Model file for the job. Use its own axes, mm. Face numbers are marked on the shaded views. A direction names the side the tool comes from. Round coordinates to 2 decimals unless told otherwise and drop trailing zeros. Loops run counter-clockwise (first coordinate to the right, second up) from the corner with the lowest first, then second, coordinate; pieces in that order, holes last. Notation, with made-up numbers: M -34.5,3.25 L -16.5,3.25 A21 cw -16.5,29.25 Z; hole C 22.25,-19 d6. An arc over 180 degrees is marked long. Use a Markdown table: item, result. Add a question column.
Item 1: Saw through at D-D on x = 30. Write the cut outline in (y, z), then the cut area to 3 significant figures.
Item 2: Saw through at C-C on z = 26. Write the cut outline in (x, y).
Item 3: Saw through at A-A on x = -22. Write the cut outline in (y, z), then the cut area to 3 significant figures.
Item 4: Saw through at B-B on y = 5.25. Give the number of separate pieces and of enclosed holes in the cut face, then the cut area to 3 significant figures.
Item 5: Pin check, flat tips, straight feed: P1, Ø2, axis at y = 6, z = 23.5, coming from the +X side; P2, Ø5, axis at x = 35, y = 1, coming from the -Z side; P3, Ø3, axis at x = 39.59, z = 45.61, coming from the -Y side; P4, Ø4.5, axis at x = 0, z = 0, coming from the +Y side. Stop position of each tip, or through.
Item 6: Tool access for the marked faces 4 and 5: list every direction of +Z, -Z, +X, -X, +Y, -Y with a clear straight run to the whole face (end or side of a thin tool).
Item 7: Two-plate mould, pull along X, no slides. Class the marked faces 1, 2 and 3: +X half, -X half, draft (parallel to the pull), parting line (faces both ways), or undercut.
Item 8: Wall check: L1, parallel to X at y = 7.5, z = 1.5; L2, parallel to Y at x = -20.5, z = -2.5; L3, parallel to X at y = 5.25, z = 45. Give the ranges that are in metal, low to high. Write a range as from..to.
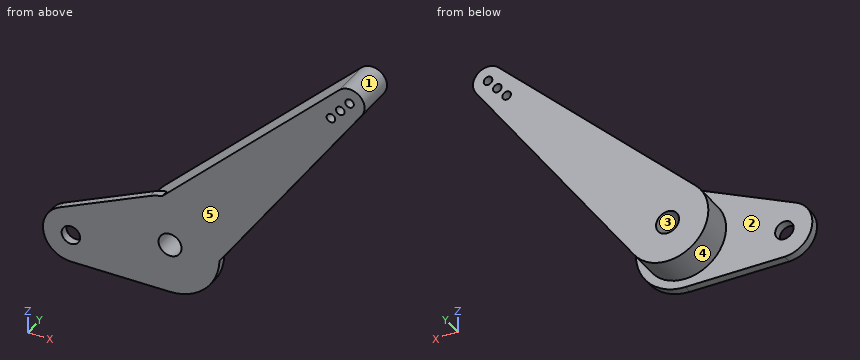
```python
from build123d import *

# Parameters (mm, degrees)
ESQUISSE1_R             = 2.675
ESQUISSE1_R_2           = 2.15
BOSS_EXTRU_1_DEPTH      = 2
BOSS_EXTRU_2_DEPTH      = 7.5
BOSS_EXTRU_2_DEPTH_BACK = 2
ESQUISSE2_R             = 2.675
ESQUISSE2_R_2           = 1


with BuildPart() as part:
    # Esquisse1 → Boss.-Extru.1 (new body)
    with BuildSketch(Plane(origin=(0, 0, 0), x_dir=(1, 0, 0), z_dir=(0, 1, 0))):
        with BuildLine():
            Line((0, 11.5), (-23.064258063, 11.5))
            ThreePointArc((-23.064258063, 11.5), (-29.416702021, 6.377118644), (-25.755971605, -0.916475151))
            Line((-25.755971605, -0.916475151), (-4.76226242, -10.467609882))
            ThreePointArc((-4.76226242, -10.467609882), (11.23893931, -2.436440678), (0, 11.5))
        make_face()
        with Locations(Location((0, 0, 0), (0, 0, 270))):
            Circle(ESQUISSE1_R, mode=Mode.SUBTRACT)
        with Locations(Location((-23.064258063, 5, 0), (0, 0, 270))):
            Circle(ESQUISSE1_R_2, mode=Mode.SUBTRACT)
    extrude(amount=BOSS_EXTRU_1_DEPTH)

    # Esquisse2 → Boss.-Extru.2 (add, two sides: drawn at the far end of the back side and taken through both)
    with BuildSketch(Plane(origin=(0, 2, 0), x_dir=(1, 0, 0), z_dir=(0, 1, 0)).offset(-BOSS_EXTRU_2_DEPTH_BACK)):
        with BuildLine():
            Line((7.728498539, 5.524519013), (44.604848398, -46.063468165))
            ThreePointArc((44.604848398, -46.063468165), (44.052017955, -50.741773707), (39.342439126, -50.632085515))
            Line((39.342439126, -50.632085515), (-6.555183772, -6.876013796))
            ThreePointArc((-6.555183772, -6.876013796), (-6.227958764, 7.173738888), (7.728498539, 5.524519013))
        make_face()
        with Locations(Location((0, 0, 0), (0, 0, 270))):
            Circle(ESQUISSE2_R, mode=Mode.SUBTRACT)
        with Locations(Location((41.757506831, -48.098817275, 0), (0, 0, 270))):
            Circle(ESQUISSE2_R_2, mode=Mode.SUBTRACT)
        with Locations(Location((39.594110629, -45.606886924, 0), (0, 0, 270))):
            Circle(ESQUISSE2_R_2, mode=Mode.SUBTRACT)
        with Locations(Location((37.430714426, -43.114956574, 0), (0, 0, 270))):
            Circle(ESQUISSE2_R_2, mode=Mode.SUBTRACT)
    extrude(amount=BOSS_EXTRU_2_DEPTH + BOSS_EXTRU_2_DEPTH_BACK)


solid = part.part
```
Entries:
| question | item | result |
|---|---|---|
| 1 | outline | M 0,25.63 L 9.5,25.63 L 9.5,41.73 L 0,41.73 Z |
| 1 | area | 153 mm2 |
| 2 | outline | M 13.5,0 L 30.26,0 L 30.26,9.5 L 13.5,9.5 Z |
| 3 | outline | M 0,-11.5 L 2,-11.5 L 2,-6.87 L 0,-6.87 Z; M 0,-3.13 L 2,-3.13 L 2,2.63 L 0,2.63 Z |
| 3 | area | 20.8 mm2 |
| 4 | separate pieces | 1 |
| 4 | enclosed holes | 4 |
| 4 | area | 961 mm2 |
| 5 | P1 | x = 29.19 |
| 5 | P2 | z = 29.13 |
| 5 | P3 | y = 0 |
| 5 | P4 | through |
| 6 | face 4 | +Y |
| 6 | face 5 | +Z, -Z, +X, -X, -Y |
| 7 | face 1 | parting line |
| 7 | face 2 | draft |
| 7 | face 3 | undercut |
| 8 | L1 | -9.38..-2.21, 2.21..12.75 |
| 8 | L2 | 0..2 |
| 8 | L3 | 33.43..38.8, 40.39..43.84 |
